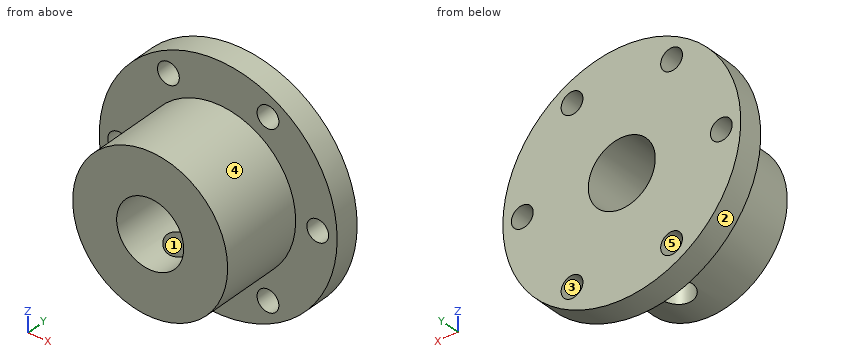
from build123d import *

# Parameters (mm, degrees)
F1_R     = 18.5
F4_DEPTH = 26.4
F2_R     = 28.4
F5_DEPTH = 6
F0_R     = 8
F6_DEPTH = 26.4
F3_R     = 2.6
F7_DEPTH = 6
F8_R     = 4
F9_DEPTH = 28


with BuildPart() as f4:
    # F1 (on Front) → F4 (new body)
    with BuildSketch(Plane.XZ):
        Circle(F1_R)
    extrude(amount=F4_DEPTH)

    # F2 (on Front) → F5 (join)
    with BuildSketch(Plane.XZ):
        Circle(F2_R)
    extrude(amount=F5_DEPTH)

    # F0 (on Front) → F6 (cut)
    with BuildSketch(Plane.XZ):
        Circle(F0_R)
    extrude(amount=F6_DEPTH, mode=Mode.SUBTRACT)

    # F3 (on Front) → F7 (cut)
    with BuildSketch(Plane.XZ):
        with Locations((-23.760727, 0)):
            Circle(F3_R)
        with Locations((-11.880363, -20.577393)):
            Circle(F3_R)
        with Locations((11.880363, -20.577393)):
            Circle(F3_R)
        with Locations((23.760727, 0)):
            Circle(F3_R)
        with Locations((11.880363, 20.577393)):
            Circle(F3_R)
        with Locations((-11.880363, 20.577393)):
            Circle(F3_R)
    extrude(amount=F7_DEPTH, mode=Mode.SUBTRACT)

    # F8 (on Top) → F9 (cut)
    with BuildSketch(Plane.XY):
        with Locations((0, -16.212996)):
            Circle(F8_R)
    extrude(amount=-F9_DEPTH, mode=Mode.SUBTRACT)


solid = f4.part
CAD build for the part. Positions are in the model's coordinates, mm. Face numbers are marked on the shaded views. A direction names the side the tool comes from. Round coordinates to 2 decimals unless told otherwise and drop trailing zeros. Write each loop counter-clockwise with the first axis right and the second up, starting at its lowest first coordinate (ties: lowest second). Pieces come first, ordered by that corner, then holes.
(1) Slice it at A-A, the plane x = 0. Write the cut outline in (y, z).
(2) Probe line 1 along Y through (x, z) = (0, -12); line 2 along X through (y, z) = (-7.75, -7); line 3 along Z through (x, y) = (-4.5, -24.25). List the from-to ranges inside material, lowest first.
(3) Drop flat-ended pins along their axis: P1, Ø6, axis at x = 23.76, z = 0, coming from the +Y side; P2, Ø5, axis at x = 10, y = -10.5, coming from the +Z side; P3, Ø7, axis at x = -11.88, z = 20.58, coming from the -Y side; P4, Ø12, axis at x = -20.5, y = -6.5, coming from the -Z side. Give the stop position or say it passes through.
(4) 3-axis set-ups, long thin cutter, end or side, ignore diameter. For the marked faces 4 and 5: which of +Z, -Z, +X, -X, +Y, -Y reach the whole face in a straight line?
(5) Mould opens along Z. For the marked faces 1, 2 and 3 say: pulls with the +Z half, pulls with the -Z half, needs draft (parallel to the pull), parting line crosses it, or undercut.
(6) Slice it at B-B, the plane z = 0. Write the cut outline in (x, y), and give its area (3 significant figures).
(7) Slice it at C-C, the plane z = 19.5. Write the cut outline in (x, y).
(8) Slice it at D-D, the plane y = -24.25. Write the cut outline in (x, z), and give its area (3 significant figures).
From the geometry:
1. outline: (-26.4, -18.5) - (-20.21, -18.5) - (-20.21, -8) - (-26.4, -8) - close; (-26.4, 8) - (0, 8) - (0, 28.4) - (-6, 28.4) - (-6, 18.5) - (-26.4, 18.5) - close; (-12.21, -18.5) - (-6, -18.5) - (-6, -28.4) - (0, -28.4) - (0, -8) - (-12.21, -8) - close
2. line 1: y = -26.4 to -20.21, -12.21 to 0
2. line 2: x = -17.12 to -3.87, 3.87 to 17.12
2. line 3: z = -17.94 to -6.61, 6.61 to 17.94
3. P1: stops at y = 0
3. P2: stops at z = 16.91
3. P3: stops at y = -6
3. P4: stops at z = -24.41
4. face 4: -Y
4. face 5: +Y, -Y
5. face 1: needs draft
5. face 2: parting line crosses it
5. face 3: undercut
6. outline: (-28.4, -6) - (-26.36, -6) - (-26.36, 0) - (-28.4, 0) - close; (-21.16, -6) - (-18.5, -6) - (-18.5, -26.4) - (-8, -26.4) - (-8, 0) - (-21.16, 0) - close; (8, -26.4) - (18.5, -26.4) - (18.5, -6) - (21.16, -6) - (21.16, 0) - (8, 0) - close; (26.36, -6) - (28.4, -6) - (28.4, 0) - (26.36, 0) - close
6. area: 611 mm2
7. outline: (-20.65, -6) - (-14.25, -6) - (-14.25, 0) - (-20.65, 0) - close; (-9.51, -6) - (9.51, -6) - (9.51, 0) - (-9.51, 0) - close; (14.25, -6) - (20.65, -6) - (20.65, 0) - (14.25, 0) - close
8. outline: circle Ø37 at (0, 0); hole circle Ø16 at (0, 0)
8. area: 874 mm2
